from build123d import *

# Parameters (mm, degrees)
SKETCH1_W           = 25.4
SKETCH1_H           = 38.1
BOSS_EXTRUDE1_DEPTH = 50.8
SHELL1_T            = -3.175
FILLET1_R           = 3.175


with BuildPart() as part:
    # Sketch1 → Boss-Extrude1 (new body)
    with BuildSketch(Plane.XY):
        Rectangle(SKETCH1_W, SKETCH1_H)
    extrude(amount=-BOSS_EXTRUDE1_DEPTH)

    # Shell1
    shell1_openings = [part.faces().sort_by_distance(p)[0] for p in [
        (0, 0, -50.8),
        (-12.7, 0, -25.4),
        (0, 19.05, -25.4),
    ]]
    offset(amount=SHELL1_T, openings=shell1_openings, kind=Kind.INTERSECTION)

    # Fillet1
    fillet1_edges = [part.edges().sort_by_distance(p)[0] for p in [
        (9.525, -15.875, -26.9875),
        (9.525, 1.5875, -3.175),
        (-1.5875, -15.875, -3.175),
    ]]
    fillet(fillet1_edges, radius=FILLET1_R)


solid = part.part
Read the model definition and answer for the solid it produces. Units are mm, in the model's axes. A direction names the side the tool comes from. Round coordinates to 2 decimals unless told otherwise and drop trailing zeros. Order: outer loops, then holes, each group sorted by start corner. A loop starts at its lowest first (then second) coordinate and runs counter-clockwise, first axis right, second up.
1) Straight lines are drawn through the part: L1, parallel to X at y = -10.5, z = -21 (3 decimals); L2, parallel to Y at x = 1.5, z = -17.5 (3 decimals); L3, parallel to Z at x = 4.5, y = -2.5 (3 decimals). For each, find the intervals that lie inside material, in ascending order.
2) The part is cut by section B-B on z = -16.5. Write down the section's boundary in (x, y) (3 decimals), plus the area to 3 significant figures.
3) For faces 1 (the face through (12.7, 0, -25)), 2 (the face through (-3.31, -14.97, -4.13)), determine the directions among +Z, -Z, +X, -X, +Y, -Y from which every point of the face is accessible in a straight line to the end or side of a thin tool.
4) Flat-ended cylindrical pins translate along their axes: pin 1 (16 mm diameter, centred on y = 7.5, z = -31, fed in from -X) (3 decimals); pin 2 (10 mm diameter, centred on x = 4, z = -16.5, fed in from +Y); pin 3 (9.5 mm diameter, centred on x = -6, z = -22, fed in from +Y) (3 decimals). Find the tip coordinate at first contact, or state that the pin passes through.
5) The part is cut by section A-A on x = 0. Write down the section's boundary in (y, z) (3 decimals), plus the area to 3 significant figures.
Resolved:
1. L1: x = 9.525 to 12.7
1. L2: y = -19.05 to -15.875
1. L3: z = -3.175 to 0
2. outline: (-12.7, -19.05) - (12.7, -19.05) - (12.7, 19.05) - (9.525, 19.05) - (9.525, -12.7) arc R3.175 cw to (6.35, -15.875) - (-12.7, -15.875) - close
2. area: 194 mm2
3. face 1: +Z, -Z, +X, +Y, -Y
3. face 2: -Z, -X, +Y
4. pin 1: stops at x = 9.525
4. pin 2: stops at y = -14.45
4. pin 3: stops at y = -15.875
5. outline: (-19.05, -50.8) - (-15.875, -50.8) - (-15.875, -6.35) arc R3.175 cw to (-12.7, -3.175) - (19.05, -3.175) - (19.05, 0) - (-19.05, 0) - close
5. area: 274 mm2
